Geometry: final body of the model. Coordinates: model frame, mm. A direction names the side the tool comes from. Give positions to 0.01 mm unless a question says otherwise; leave off trailing zeros. Write each loop counter-clockwise with the first axis right and the second up, starting at its lowest first coordinate (ties: lowest second). Pieces come first, ordered by that corner, then holes. Notation, with made-up numbers: M 67.25,-23.5 L 99.25,-23.5 A24 cw 99.25,13.5 Z; hole C 44.5,22.5 d3. An arc over 180 degrees is marked long. Answer as a JSON object with one key per item and string values.
from build123d import *

# Parameters (mm, degrees)
BOSS_EXTRUDE1_DEPTH = 10


with BuildPart() as part:
    # Sketch1 → Boss-Extrude1 (new body)
    with BuildSketch(Plane.XY):
        with BuildLine():
            Line((26.73180705, 202.268045215), (-266.122767511, 202.268045215))
            Line((-266.122767511, 202.268045215), (-267.623671515, 191.109569167))
            Line((-267.623671515, 191.109569167), (-273.353298876, 182.913754973))
            Line((-273.353298876, 182.913754973), (-231.718562767, 153.807247983))
            Line((-231.718562767, 153.807247983), (-225.988935407, 162.003062177))
            Line((-225.988935407, 162.003062177), (-184.354199298, 132.896555187))
            Line((-184.354199298, 132.896555187), (-190.083826658, 124.700740993))
            Line((-190.083826658, 124.700740993), (-148.449090549, 95.594234003))
            Line((-148.449090549, 95.594234003), (-142.719463189, 103.790048198))
            Line((-142.719463189, 103.790048198), (-101.084727081, 74.683541208))
            Line((-101.084727081, 74.683541208), (-106.814354441, 66.487727013))
            Line((-106.814354441, 66.487727013), (-65.179618332, 37.381220023))
            Line((-65.179618332, 37.381220023), (-59.449990972, 45.577034218))
            Line((-59.449990972, 45.577034218), (-17.815254863, 16.470527228))
            Line((-17.815254863, 16.470527228), (-23.544882223, 8.274713033))
            Line((-23.544882223, 8.274713033), (-23.544882223, -182.686538243))
            Line((-23.544882223, -182.686538243), (496.44897172, -182.686538243))
            Line((496.44897172, -182.686538243), (496.44897172, -32.421529871))
            ThreePointArc((496.44897172, -32.421529871), (474.130508447, 21.460006856), (420.24897172, 43.778470129))
            Line((420.24897172, 43.778470129), (253.439588816, 43.778470129))
            Line((253.439588816, 43.778470129), (26.73180705, 202.268045215))
        make_face()
        Polygon((23.819481246, -12.635979762), (65.454217354, -41.742486752), (59.724589994, -49.938300947), (18.089853885, -20.831793957), align=None, mode=Mode.SUBTRACT)
        Polygon((107.088953463, -70.848993742), (148.723689572, -99.955500732), (142.994062212, -108.151314927), (101.359326103, -79.044807937), align=None, mode=Mode.SUBTRACT)
        Polygon((190.358425681, -129.062007722), (231.993161789, -158.168514712), (226.263534429, -166.364328907), (184.62879832, -137.257821917), align=None, mode=Mode.SUBTRACT)
        Polygon((299.480024398, -151.692530547), (345.520459979, -130.22352285), (349.746642597, -139.28660072), (303.706207015, -160.755608417), align=None, mode=Mode.SUBTRACT)
        Polygon((391.560895561, -108.754515154), (437.601331142, -87.285507457), (441.82751376, -96.348585328), (395.787078178, -117.817593024), align=None, mode=Mode.SUBTRACT)
    extrude(amount=BOSS_EXTRUDE1_DEPTH)


solid = part.part
1) Cut plane B-B on z = 8.25. Give the number of separate pieces and of enclosed holes in the cut face, and give its area (3 significant figures).
Geometry check:
{"separate pieces": "1", "enclosed holes": "5", "area": "165,000 mm2"}
2) Line query: line 1 (X direction, y = -52.5, z = 3.5); line 2 (X direction, y = 157, z = 1.75); line 3 (Y direction, x = 147, z = 2). Output: solid intervals per line, ascending. Write a range as from..to.
Geometry check:
{"line 1": "x = -23.54..496.45", "line 2": "x = -236.29..-229.49, -218.83..91.48", "line 3": "y = -182.69..-102.42, -98.75..118.19"}
3) Cut plane D-D on y = 82. Return loops of the section in (x, z), and give its area (3 significant figures).
Geometry check:
{"outline": "M -111.55,0 L 198.77,0 L 198.77,10 L -111.55,10 Z", "area": "3,100 mm2"}
4) Pull-direction query (X, two-part tool) for faces 3 (the flat face through (106, 12, 10)), 4 (the flat face through (327.05, -149.87, 4.93)), 5 (the flat face through (-169.558, 110.351, 4.93)); classes: pulls with the +X half, pulls with the -X half, needs draft (parallel to the pull), parting line crosses it, or undercut.
Geometry check:
{"face 3": "needs draft", "face 4": "undercut", "face 5": "pulls with the -X half"}
5) Cut plane C-C on x = 117. Return loops of the section in (y, z), and give its area (3 significant figures).
Geometry check:
{"outline": "M -182.69,0 L -89.98,0 L -89.98,10 L -182.69,10 Z; M -77.78,0 L 139.16,0 L 139.16,10 L -77.78,10 Z", "area": "3,100 mm2"}
6) Contact query for flat-ended pins moving along their axis: P1, Ø5, axis at x = 358.5, z = 3, coming from the +Y side; P2, Ø5, axis at y = -0.5, z = 1.5, coming from the +X side; P3, Ø3, axis at y = -122.5, z = 6, coming from the -X side. Output: stop coordinate, or through.
Geometry check:
{"P1": "stops at y = 43.78", "P2": "stops at x = 490.54", "P3": "stops at x = -23.54"}
7) Cut plane A-A on x = 330. Return loops of the section in (y, z).
Geometry check:
{"outline": "M -182.69,0 L -148.49,0 L -148.49,10 L -182.69,10 Z; M -137.46,0 L 43.78,0 L 43.78,10 L -137.46,10 Z"}
8) Set-up query: faces 1 (the flat face through (419.13, -106.933, 4.93)), 2 (the flat face through (-252.827, 168.564, 4.93)). Return all of +Z, -Z, +X, -X, +Y, -Y with unobstructed straight access to the full face (end or side cutting, diameter ignored); none if empty.
Geometry check:
{"face 1": "+Z, -Z", "face 2": "+Z, -Z, -X, -Y"}
